Build history of the part. All positions in model axes, mm. Face numbers are marked on the shaded views. Coordinates: 2 decimals unless noted, no trailing zeros. Write each loop counter-clockwise with the first axis right and the second up, starting at its lowest first coordinate (ties: lowest second). Pieces come first, ordered by that corner, then holes.
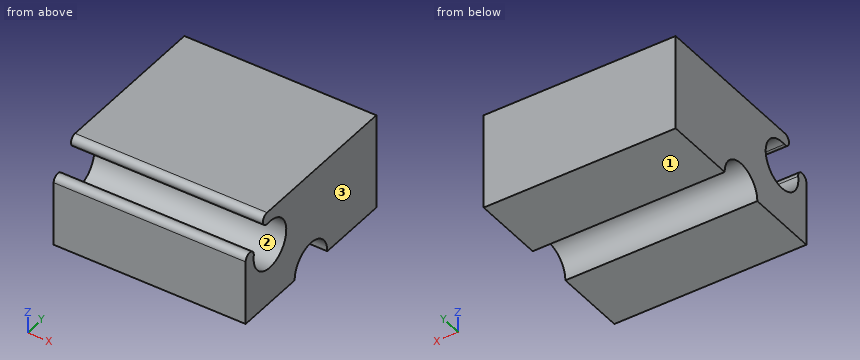
```python
from build123d import *

# Parameters (mm, degrees)
F1_DEPTH = 25.4


with BuildPart() as f1:
    # F0 (on Right) → F1 (new body, symmetric)
    with BuildSketch(Plane.YZ):
        with BuildLine():
            ThreePointArc((-0.898026, 6.286179), (4.490128, -4.490128), (-6.286179, 0.898026))
            ThreePointArc((-6.286179, 0.898026), (-7.745188, 2.706038), (-9.445224, 1.122532))
            Line((-9.445224, 1.122532), (-9.445224, -15.954776))
            Line((-9.445224, -15.954776), (9.604776, -15.954776))
            ThreePointArc((9.604776, -15.954776), (15.954776, -9.604776), (22.304776, -15.954776))
            Line((22.304776, -15.954776), (41.354776, -15.954776))
            Line((41.354776, -15.954776), (41.354776, 9.445224))
            Line((41.354776, 9.445224), (-1.122532, 9.445224))
            ThreePointArc((-1.122532, 9.445224), (-2.706038, 7.745188), (-0.898026, 6.286179))
        make_face()
    extrude(amount=F1_DEPTH, both=True)


solid = f1.part
```
1. Saw through at B-B on z = 0. List the corners of the cut face in (x, y).
Computed values:
outline: (-25.4, -9.45) - (25.4, -9.45) - (25.4, -6.35) - (-25.4, -6.35) - close; (-25.4, 6.35) - (25.4, 6.35) - (25.4, 41.35) - (-25.4, 41.35) - close
2. Flat gauge pins, fed straight in: pin 1 (11.5 mm diameter, centred on y = 0, z = 0, fed in from -X); pin 2 (3 mm diameter, centred on x = -16.5, y = 17, fed in from -Z). Where does each tip first touch, or does it go through?
Computed values:
pin 1: passes through
pin 2: stops at z = -10.14
3. Saw through at A-A on y = 0. List the corners of the cut face in (x, z).
Computed values:
outline: (-25.4, -15.95) - (25.4, -15.95) - (25.4, -6.35) - (-25.4, -6.35) - close; (-25.4, 6.35) - (25.4, 6.35) - (25.4, 9.45) - (-25.4, 9.45) - close
4. Saw through at D-D on z = 4. List the corners of the cut face in (x, y), plus the area to 3 significant figures.
Computed values:
outline: (-25.4, 4.93) - (25.4, 4.93) - (25.4, 41.35) - (-25.4, 41.35) - close
area: 1,850 mm2
5. Mould opens along Z. For the marked faces 1, 2 and 3 say: +Z half, -Z half, draft (parallel to the pull), parting line (faces both ways), or undercut.
Computed values:
face 1: -Z half
face 2: undercut
face 3: draft
6. Probe line 1 along Y through (x, z) = (-14, 0); line 2 along Z through (x, y) = (-12, 0); line 3 along Z through (x, y) = (-17.5, 16). List the from-to ranges inside material, lowest first.
Computed values:
line 1: y = -9.45 to -6.35, 6.35 to 41.35
line 2: z = -15.95 to -6.35, 6.35 to 9.45
line 3: z = -9.6 to 9.45
